Read the model definition and answer for the solid it produces. Units are mm, in the model's axes. Face numbers are marked on the shaded views. Coordinates: 2 decimals unless noted, no trailing zeros. Write each loop counter-clockwise with the first axis right and the second up, starting at its lowest first coordinate (ties: lowest second). Pieces come first, ordered by that corner, then holes.
(1) Section D-D on z = 39 is taken. Write down the section's boundary in (x, y).
(2) Section A-A on x = 0 is taken. Write down the section's boundary in (y, z).
(3) The mould has two halves that part along X. Classify the marked faces 1, 2, 3 and 4: +X half, -X half, draft (parallel to the pull), parting line (faces both ways), or undercut.
(4) Find the intervals of material crossed by probe 1 along Z at (x, y) = (0, 13); probe 2 along Z at (x, y) = (-9, 1.5); probe 3 along X at (y, z) = (10.5, -23.5), in increasing order.
(5) Given pin 1 (1 mm diameter, centred on x = 32.5, y = 3, fed in from +Z); pin 2 (12 mm diameter, centred on x = 46, y = 7, fed in from -Z); pin 3 (4 mm diameter, centred on y = 19.5, z = 13, fed in from -X), each flat-ended and moving along its own axis, determine where each tip first touches the part or whether it passes through.
(6) Section C-C on x = 15 is taken. Write down the section's boundary in (y, z), then the cut area to 3 significant figures.
(7) Section B-B on y = 2.5 is taken. Write down the section's boundary in (x, z), then the cut area to 3 significant figures.
from build123d import *

# Parameters (mm, degrees)
SKETCH1_R           = 10
SKETCH1_R_2         = 5
BOSS_EXTRUDE1_DEPTH = 30


with BuildPart() as part:
    # Sketch1 → Boss-Extrude1 (new body)
    with BuildSketch(Plane(origin=(0, 0, 0), x_dir=(1, 0, 0), z_dir=(0, 1, 0))):
        with BuildLine():
            Line((-15, 24.031639244), (-10, -19.968360756))
            ThreePointArc((-10, -19.968360756), (0, -29.968360756), (10, -19.968360756))
            ThreePointArc((10, -19.968360756), (29.477373415, -18.829083409), (47.176676653, -27.038875908))
            Line((47.176676653, -27.038875908), (86.964311464, -59.258267297))
            Line((86.964311464, -59.258267297), (93.257515375, -51.486807682))
            ThreePointArc((93.257515375, -51.486807682), (83.004155911, -32.566658766), (77.036161898, -11.890913004))
            Line((77.036161898, -11.890913004), (8.638834838, 36.294205559))
            ThreePointArc((8.638834838, 36.294205559), (-6.907151274, 37.346715709), (-15, 24.031639244))
        make_face()
        with Locations((0, 24.031639244)):
            Circle(SKETCH1_R, mode=Mode.SUBTRACT)
        with Locations((0, -19.968360756)):
            Circle(SKETCH1_R_2, mode=Mode.SUBTRACT)
    extrude(amount=BOSS_EXTRUDE1_DEPTH)


solid = part.part
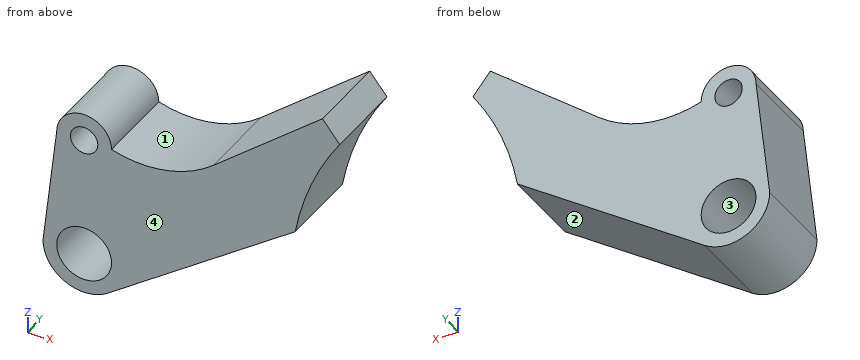
Response:
1. outline: (61.95, 0) - (85.91, 0) - (85.91, 30) - (61.95, 30) - close
2. outline: (0, -39.03) - (30, -39.03) - (30, -34.03) - (0, -34.03) - close; (0, -14.03) - (30, -14.03) - (30, 14.97) - (0, 14.97) - close; (0, 24.97) - (30, 24.97) - (30, 29.97) - (0, 29.97) - close
3. face 1: undercut
3. face 2: +X half
3. face 3: undercut
3. face 4: draft
4. probe 1: z = -39.03 to -34.03, -14.03 to 14.97, 24.97 to 29.97
4. probe 2: z = -36.03 to -28.39, -19.67 to 24.33
4. probe 3: x = -14.94 to -9.99, 9.99 to 26.8
5. pin 1: stops at z = 19.67
5. pin 2: stops at z = -14.2
5. pin 3: stops at x = -11.02
6. outline: (0, -31.81) - (30, -31.81) - (30, 18.74) - (0, 18.74) - close
6. area: 1,520 mm2
7. outline: (-15, -24.03) arc R15 ccw to (8.64, -36.29) - (77.04, 11.89) arc R100 cw to (93.26, 51.49) - (86.96, 59.26) - (47.18, 27.04) arc R40 cw to (10, 19.97) arc R10 ccw to (-10, 19.97) - close; hole circle Ø20 at (0, -24.03); hole circle Ø10 at (0, 19.97)
7. area: 4,090 mm2
